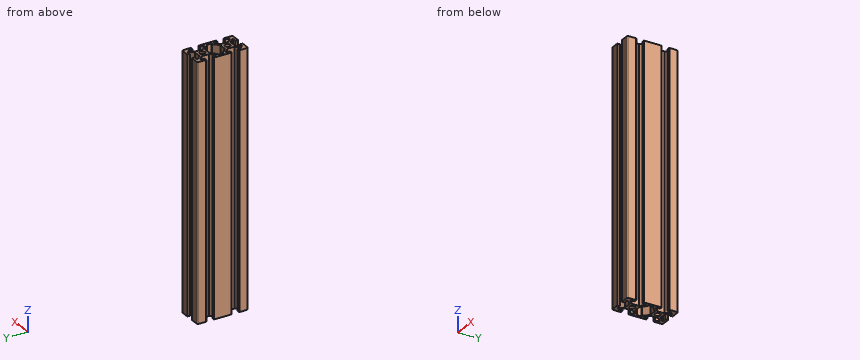
```python
from build123d import *

# Parameters (mm, degrees)
SKETCH1_R           = 2.1
BOSS_EXTRUDE1_DEPTH = 200
FILLET1_R           = 0.1


with BuildPart() as part:
    # Sketch1 → Boss-Extrude1 (new body)
    with BuildSketch(Plane.XY):
        with BuildLine():
            Line((10, -19), (10, -13))
            Line((10, -13), (8, -13))
            Line((8, -13), (8, -16))
            Line((8, -16), (7, -16))
            Line((7, -16), (4, -13))
            Line((4, -13), (4, -7))
            Line((4, -7), (7, -4))
            Line((7, -4), (8, -4))
            Line((8, -4), (8, -7))
            Line((8, -7), (10, -7))
            Line((10, -7), (10, 7))
            Line((10, 7), (8, 7))
            Line((8, 7), (8, 4))
            Line((8, 4), (7, 4))
            Line((7, 4), (4, 7))
            Line((4, 7), (4, 13))
            Line((4, 13), (7, 16))
            Line((7, 16), (8, 16))
            Line((8, 16), (8, 13))
            Line((8, 13), (10, 13))
            Line((10, 13), (10, 19))
            ThreePointArc((10, 19), (9.707106781, 19.707106781), (9, 20))
            Line((9, 20), (3, 20))
            Line((3, 20), (3, 18))
            Line((3, 18), (6, 18))
            Line((6, 18), (6, 17))
            Line((6, 17), (3, 14))
            Line((3, 14), (-3, 14))
            Line((-3, 14), (-6, 17))
            Line((-6, 17), (-6, 18))
            Line((-6, 18), (-3, 18))
            Line((-3, 18), (-3, 20))
            Line((-3, 20), (-9, 20))
            ThreePointArc((-9, 20), (-9.707106781, 19.707106781), (-10, 19))
            Line((-10, 19), (-10, 13))
            Line((-10, 13), (-8, 13))
            Line((-8, 13), (-8, 16))
            Line((-8, 16), (-7, 16))
            Line((-7, 16), (-4, 13))
            Line((-4, 13), (-4, 7))
            Line((-4, 7), (-7, 4))
            Line((-7, 4), (-8, 4))
            Line((-8, 4), (-8, 7))
            Line((-8, 7), (-10, 7))
            Line((-10, 7), (-10, -7))
            Line((-10, -7), (-8, -7))
            Line((-8, -7), (-8, -4))
            Line((-8, -4), (-7, -4))
            Line((-7, -4), (-4, -7))
            Line((-4, -7), (-4, -13))
            Line((-4, -13), (-7, -16))
            Line((-7, -16), (-8, -16))
            Line((-8, -16), (-8, -13))
            Line((-8, -13), (-10, -13))
            Line((-10, -13), (-10, -19))
            ThreePointArc((-10, -19), (-9.707106781, -19.707106781), (-9, -20))
            Line((-9, -20), (-3, -20))
            Line((-3, -20), (-3, -18))
            Line((-3, -18), (-6, -18))
            Line((-6, -18), (-6, -17))
            Line((-6, -17), (-3, -14))
            Line((-3, -14), (3, -14))
            Line((3, -14), (6, -17))
            Line((6, -17), (6, -18))
            Line((6, -18), (3, -18))
            Line((3, -18), (3, -20))
            Line((3, -20), (9, -20))
            ThreePointArc((9, -20), (9.707106781, -19.707106781), (10, -19))
        make_face()
        with Locations((0, -10)):
            Circle(SKETCH1_R, mode=Mode.SUBTRACT)
        with Locations((0, 10)):
            Circle(SKETCH1_R, mode=Mode.SUBTRACT)
        Polygon((-7, -2), (-8, -2), (-8, 2), (-7, 2), (-3, 6), (3, 6), (7, 2), (8, 2), (8, -2), (7, -2), (3, -6), (-3, -6), align=None, mode=Mode.SUBTRACT)
    extrude(amount=-BOSS_EXTRUDE1_DEPTH)

    # Fillet1
    fillet1_edges = [part.edges().sort_by_distance(p)[0] for p in [
        (-10, -13, -100),
        (-10, -7, -100),
        (-10, 7, -100),
        (-10, 13, -100),
        (10, 13, -100),
        (10, 7, -100),
        (10, -7, -100),
        (10, -13, -100),
    ]]
    fillet(fillet1_edges, radius=FILLET1_R)


solid = part.part
```
Here's how the part is built. I have some questions about the finished solid (model axes, mm). Round coordinates to 2 decimals unless told otherwise and drop trailing zeros. Order: outer loops, then holes, each group sorted by start corner. A loop starts at its lowest first (then second) coordinate and runs counter-clockwise, first axis right, second up. Notation, with made-up numbers: (-13, -32.75) -> (-1, -32.75) arc R18 ccw to (-1, 1.25) -> close; hole circle Ø6 at (51.25, 75). An arc over 180 degrees is marked (long way). Use a Markdown table: item, result. Add a question column.
(1) Suppose I cut it at B-B, the plane z = -35. Count the separate pieces of the cut face and the enclosed holes in it, and give its area (3 significant figures).
(2) Suppose I cut it at A-A, the plane y = 10. Please give me the cut outline in (x, z).
(3) I need wall thicknesses on line 1 along Y through (x, z) = (-7, -99.5); line 2 along Y through (x, z) = (0, -129.5); line 3 along X through (y, z) = (15, -78). Which ranges of each line are inside material? Lowest first, please.
(4) For pin 1 Ø1.8 at (y, z) = (9.5, -112.5) entering from +X; pin 2 Ø1.8 at (y, z) = (11, -52) entering from -X, each with a flat end and sliding along its axis, tell me the tip position at first contact or that it passes through.
Verdict:
| question | item | result |
|---|---|---|
| 1 | separate pieces | 1 |
| 1 | enclosed holes | 3 |
| 1 | area | 321 mm2 |
| 2 | outline | (-4, -200) -> (-2.1, -200) -> (-2.1, 0) -> (-4, 0) -> close; (2.1, -200) -> (4, -200) -> (4, 0) -> (2.1, 0) -> close |
| 3 | line 1 | -20 to -16, -4 to -2, 2 to 4, 16 to 20 |
| 3 | line 2 | -14 to -12.1, -7.9 to -6, 6 to 7.9, 12.1 to 14 |
| 3 | line 3 | -10 to -8, -6 to -4, 4 to 6, 8 to 10 |
| 4 | pin 1 | x = 4 |
| 4 | pin 2 | x = -4 |
